Geometry check sheet. Reference: the model listing, model coordinates, mm. A direction names the side the tool comes from. Round coordinates to 2 decimals unless told otherwise and drop trailing zeros. Write each loop counter-clockwise with the first axis right and the second up, starting at its lowest first coordinate (ties: lowest second). Pieces come first, ordered by that corner, then holes. Notation, with made-up numbers: M 75.5,53 L 99.5,53 A5 cw 99.5,62 Z; hole C -19,1.5 d9. An arc over 180 degrees is marked long. Use a Markdown table: item, result.
```python
from build123d import *

# Parameters (mm, degrees)
SZKIC1_R                    = 9
DODANIE_WYCI_GNI_CIE1_DEPTH = 166
SZKIC2_R                    = 9.5
DODANIE_WYCI_GNI_CIE2_DEPTH = 175
SZKIC3_R                    = 17.5
DODANIE_WYCI_GNI_CIE3_DEPTH = 36
SFAZOWANIE1_SIZE            = 5
WYTNIJ_WYCI_GNI_CIE1_START  = -10
SZKIC8_R                    = 9
WYTNIJ_WYCI_GNI_CIE1_DEPTH  = 10
SFAZOWANIE3_SIZE            = 3.5
SFAZOWANIE1_OF_LUSTRO7_SIZE = 5
SFAZOWANIE3_OF_LUSTRO7_SIZE = 3.5


with BuildPart() as part:
    # Szkic1 → Dodanie-wyciągnięcie1 (new body)
    with BuildSketch(Plane(origin=(0, 0, 0), x_dir=(0, 0, -1), z_dir=(1, 0, 0))):
        Circle(SZKIC1_R)
    extrude(amount=DODANIE_WYCI_GNI_CIE1_DEPTH)

    # Szkic2 → Dodanie-wyciągnięcie2 (add)
    with BuildSketch(Plane.ZY):
        Circle(SZKIC2_R)
    extrude(amount=DODANIE_WYCI_GNI_CIE2_DEPTH)

    # Szkic3 → Dodanie-wyciągnięcie3 (add)
    with BuildSketch(Plane(origin=(166, 0, 0), x_dir=(0, 0, -1), z_dir=(1, 0, 0))):
        Circle(SZKIC3_R)
    dodanie_wyci_gni_cie3 = extrude(amount=DODANIE_WYCI_GNI_CIE3_DEPTH)

    # Sfazowanie1
    sfazowanie1_edges = [part.edges().sort_by_distance(p)[0] for p in [
        (202, 0, 17.5),
    ]]
    chamfer(sfazowanie1_edges, length=SFAZOWANIE1_SIZE)

    # Szkic8 → Wytnij-wyciągnięcie1 (cut)
    with BuildSketch(Plane(origin=(202, 0, 0), x_dir=(0, 0, -1), z_dir=(1, 0, 0)).offset(WYTNIJ_WYCI_GNI_CIE1_START)):
        Circle(SZKIC8_R)
    wytnij_wyci_gni_cie1 = extrude(amount=WYTNIJ_WYCI_GNI_CIE1_DEPTH, mode=Mode.SUBTRACT)

    # Szkic4 → Wycięcie-obrót9 (revolve, cut)
    with BuildSketch(Plane.XY):
        with BuildLine():
            Line((189.5, 12.5), (189.5, -12.5))
            ThreePointArc((189.5, -12.5), (202, 0), (189.5, 12.5))
        make_face()
    wyci_cie_obr_t9 = revolve(axis=Axis((189.5, 12.5, 0), (0, -1, 0)), mode=Mode.SUBTRACT)

    # Sfazowanie3
    sfazowanie3_edges = [part.edges().sort_by_distance(p)[0] for p in [
        (202, 0, 9),
    ]]
    chamfer(sfazowanie3_edges, length=SFAZOWANIE3_SIZE - 0.0001)  # a hair under: the kernel refuses the full size

    # Lustro7: Dodanie-wyciągnięcie3, Wytnij-wyciągnięcie1, Wycięcie-obrót9 across plane
    add(dodanie_wyci_gni_cie3.mirror(Plane.ZY.offset(4.5)))
    add(wytnij_wyci_gni_cie1.mirror(Plane.ZY.offset(4.5)), mode=Mode.SUBTRACT)
    add(wyci_cie_obr_t9.mirror(Plane.ZY.offset(4.5)), mode=Mode.SUBTRACT)

    # Sfazowanie1 of Lustro7
    sfazowanie1_of_lustro7_edges = [part.edges().sort_by_distance(p)[0] for p in [
        (-211, 0, 17.5),
    ]]
    chamfer(sfazowanie1_of_lustro7_edges, length=SFAZOWANIE1_OF_LUSTRO7_SIZE)

    # Sfazowanie3 of Lustro7
    sfazowanie3_of_lustro7_edges = [part.edges().sort_by_distance(p)[0] for p in [
        (-211, 0, 9),
    ]]
    chamfer(sfazowanie3_of_lustro7_edges, length=SFAZOWANIE3_OF_LUSTRO7_SIZE - 0.0001)  # a hair under: the kernel refuses the full size


solid = part.part
```
Item 1: Mould release check, pull along X, two halves, no side actions. Record for faces 5 (the face through (-207.67, -3.51, -8.47)), 6 (the face through (-86.28, -8.43, 4.38)), 7 (the face through (181.283, -10.648, 13.887)): +X half, -X half, draft (parallel to the pull), parting line (faces both ways), or undercut.
Outcome:
| item | result |
|---|---|
| face 5 | -X half |
| face 6 | undercut |
| face 7 | draft |
Item 2: Access from +Z, -Z, +X, -X, +Y, -Y to the whole of each face (thin tool, end or side, straight path). Record for faces 1 (the face through (-175, -8, -8)), 2 (the face through (-207.335, 8.923, 1.172)), 3 (the face through (-190.283, -10.648, 13.887)), 4 (the face through (198.335, 8.923, 1.172)).
Outcome:
| item | result |
|---|---|
| face 1 | none |
| face 2 | -X |
| face 3 | +X, -X |
| face 4 | +X |
Item 3: Material ranges on line 1 along X through (y, z) = (-11, -11.5); line 2 along X through (y, z) = (10.5, -3.5); line 3 along X through (y, z) = (-8, 12.5), recorded low to high. Write a range as from..to.
Outcome:
| item | result |
|---|---|
| line 1 | x = -207.59..-175, 166..198.59 |
| line 2 | x = -209.57..-204.31, -192.69..-175, 166..183.69, 195.31..200.57 |
| line 3 | x = -208.66..-175, 166..199.66 |
Item 4: Cross-section at D-D, the plane x = 88.5. Record the cut outline in (y, z), and give its area (3 significant figures).
Outcome:
| item | result |
|---|---|
| outline | C 0,0 d18 |
| area | 254 mm2 |
Item 5: Go/stop test with flat-tipped pins: pin 1 (1 mm diameter, centred on y = -2.5, z = -4, fed in from +X); pin 2 (2 mm diameter, centred on x = 38.5, z = 7.5, fed in from -Y); pin 3 (1.5 mm diameter, centred on x = 50.5, y = -4, fed in from -Z). Record where each tip stops, or that it passes through.
Outcome:
| item | result |
|---|---|
| pin 1 | stops at x = 178.14 |
| pin 2 | stops at y = -6.22 |
| pin 3 | stops at z = -8.39 |
Item 6: Cross-section at C-C, the plane x = -80.5. Record the cut outline in (y, z), and give its area (3 significant figures).
Outcome:
| item | result |
|---|---|
| outline | C 0,0 d19 |
| area | 284 mm2 |
